Design review of the part built by this model. Coordinates are the model's own, in mm. Face numbers are marked on the shaded views. Coordinates: 2 decimals unless noted, no trailing zeros. Loops run counter-clockwise (first coordinate to the right, second up) from the corner with the lowest first, then second, coordinate; pieces in that order, holes last. Notation, with made-up numbers: (-28.75, 56.25) - (-16.75, 56.25) arc R33 cw to (-16.75, 86.25) - close; hole circle Ø8 at (-12, 46.5). An arc over 180 degrees is marked (long way). Use one line per item in the form item = value. Start each with the question number.
(1) Add section A-A (x = 34.5). State the section outline as (y, z) points.
(2) Add section B-B (z = -11). State the section outline as (x, y) points, plus the area to 3 significant figures.
(3) Clearance check with flat-ended pins moving along their axes: pin 1 Ø1.5 at (y, z) = (1, 3.5) entering from -X; pin 2 Ø2 at (y, z) = (1.5, -18.5) entering from +X; pin 3 Ø2 at (x, z) = (20, -1) entering from +Y. State where each tip first meets the part, or that it passes through.
(4) For L1, parallel to X at y = 0.5, z = -39.5; L2, parallel to X at y = 1.75, z = -16; L3, parallel to Y at x = 17, z = 2, list the stretches that pass through material, from the lowest coordinate up.
(5) The part is to be moulded in two halves that separate along X. For the marked faces 1 and 2, say which applies: pulls with the +X half, pulls with the -X half, needs draft (parallel to the pull), parting line crosses it, or undercut.
(6) Add section D-D (x = 4). State the section outline as (y, z) points, plus the area to 3 significant figures.
(7) Add section C-C (y = 2.75). State the section outline as (x, z) points (3 decimals).
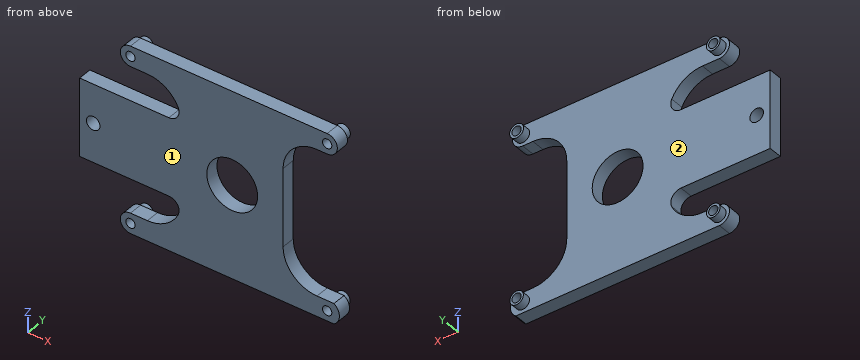
```python
from build123d import *

# Parameters (mm, degrees)
SKETCH2_R           = 1.375
SKETCH2_R_2         = 7.5
BOSS_EXTRUDE1_DEPTH = 4
SKETCH3_R           = 2
CUT_EXTRUDE1_DEPTH  = 10
SKETCH7_R           = 1.995105634
SKETCH7_R_2         = 1.375
SKETCH7_R_3         = 2.001880143
SKETCH7_R_4         = 2.050219115
SKETCH7_R_5         = 2.002328612
BOSS_EXTRUDE2_DEPTH = 2.4


with BuildPart() as part:
    # Sketch2 → Boss-Extrude1 (new body)
    with BuildSketch(Plane(origin=(0, 0, 0), x_dir=(1, 0, 0), z_dir=(0, 1, 0))):
        with BuildLine():
            Line((43.240356283, 42.558742845), (-16.759643717, 42.558742845))
            ThreePointArc((-16.759643717, 42.558742845), (-19.759643717, 39.558742845), (-16.759643717, 36.558742845))
            Line((-16.759643717, 36.558742845), (-11.759643717, 36.558742845))
            ThreePointArc((-11.759643717, 36.558742845), (-6.414418879, 35.010285392), (-2.724564688, 30.84445713))
            ThreePointArc((-2.724564688, 30.84445713), (-2.899625633, 27.955175393), (-5.435088397, 26.558742845))
            Line((-5.435088397, 26.558742845), (-28.759643717, 26.558742845))
            Line((-28.759643717, 26.558742845), (-31.759643717, 26.558742845))
            Line((-31.759643717, 26.558742845), (-31.759643717, 23.558742845))
            Line((-31.759643717, 23.558742845), (-31.759643717, 6.558742845))
            Line((-31.759643717, 6.558742845), (-31.759643717, 3.558742845))
            Line((-31.759643717, 3.558742845), (-28.759643717, 3.558742845))
            Line((-28.759643717, 3.558742845), (-5.435088397, 3.558742845))
            ThreePointArc((-5.435088397, 3.558742845), (-2.899625633, 2.162310296), (-2.724564688, -0.726971441))
            ThreePointArc((-2.724564688, -0.726971441), (-6.414418879, -4.892799703), (-11.759643717, -6.441257155))
            Line((-11.759643717, -6.441257155), (-16.759643717, -6.441257155))
            ThreePointArc((-16.759643717, -6.441257155), (-19.759643717, -9.441257155), (-16.759643717, -12.441257155))
            Line((-16.759643717, -12.441257155), (41.240356283, -12.441257155))
            ThreePointArc((41.240356283, -12.441257155), (44.240356283, -9.441257155), (41.240356283, -6.441257155))
            Line((41.240356283, -6.441257155), (38.240356283, -6.441257155))
            ThreePointArc((38.240356283, -6.441257155), (31.169288471, -3.512324967), (28.240356283, 3.558742845))
            Line((28.240356283, 3.558742845), (28.240356283, 26.558742845))
            ThreePointArc((28.240356283, 26.558742845), (31.169288471, 33.629810657), (38.240356283, 36.558742845))
            Line((38.240356283, 36.558742845), (43.240356283, 36.558742845))
            ThreePointArc((43.240356283, 36.558742845), (44.845907558, 39.558742845), (43.240356283, 42.558742845))
        make_face()
        with Locations((-16.759643717, -9.441257155)):
            Circle(SKETCH2_R, mode=Mode.SUBTRACT)
        with Locations((41.240356283, -9.441257155)):
            Circle(SKETCH2_R, mode=Mode.SUBTRACT)
        with Locations((13.240356283, 15.058742845)):
            Circle(SKETCH2_R_2, mode=Mode.SUBTRACT)
        with Locations((-16.759643717, 39.558742845)):
            Circle(SKETCH2_R, mode=Mode.SUBTRACT)
        with Locations((41.240356283, 39.558742845)):
            Circle(SKETCH2_R, mode=Mode.SUBTRACT)
    extrude(amount=BOSS_EXTRUDE1_DEPTH)

    # Sketch3 → Cut-Extrude1 (cut)
    with BuildSketch(Plane(origin=(0, 4, 0), x_dir=(1, 0, 0), z_dir=(0, 1, 0))):
        with Locations((-27.759643717, 15.058742845)):
            Circle(SKETCH3_R)
    extrude(amount=-CUT_EXTRUDE1_DEPTH, mode=Mode.SUBTRACT)

    # Sketch7 → Boss-Extrude2 (add)
    with BuildSketch(Plane(origin=(0, 4, 0), x_dir=(1, 0, 0), z_dir=(0, 1, 0))):
        with Locations((-16.759643717, 39.558742845)):
            Circle(SKETCH7_R)
        with Locations((-16.759643717, 39.558742845)):
            Circle(SKETCH7_R_2, mode=Mode.SUBTRACT)
        with Locations((-16.759643717, -9.441257155)):
            Circle(SKETCH7_R_3)
        with Locations((-16.759643717, -9.441257155)):
            Circle(SKETCH7_R_2, mode=Mode.SUBTRACT)
        with Locations((41.240356283, -9.441257155)):
            Circle(SKETCH7_R_4)
        with Locations((41.240356283, -9.441257155)):
            Circle(SKETCH7_R_2, mode=Mode.SUBTRACT)
        with Locations((41.240356283, 39.558742845)):
            Circle(SKETCH7_R_5)
        with Locations((41.240356283, 39.558742845)):
            Circle(SKETCH7_R_2, mode=Mode.SUBTRACT)
    extrude(amount=BOSS_EXTRUDE2_DEPTH)


solid = part.part
```
Computed values:
q1.outline = (0, -42.56) - (4, -42.56) - (4, -35.83) - (0, -35.83) - close; (0, 5.72) - (4, 5.72) - (4, 12.44) - (0, 12.44) - close
q2.outline = (-31.76, 0) - (6.93, 0) - (6.93, 4) - (-31.76, 4) - close; (19.55, 0) - (28.24, 0) - (28.24, 4) - (19.55, 4) - close
q2.area = 190 mm^2
q3.pin_1 = -5.51
q3.pin_2 = 28.24
q3.pin_3 = 4
q4.L1 = -19.76 to -18.13, -15.39 to 39.87, 42.61 to 44.85
q4.L2 = -31.76 to -29.52, -25.99 to 5.8, 20.68 to 28.24
q4.L3 = 0 to 4
q5.face_1 = needs draft
q5.face_2 = undercut
q6.outline = (0, -42.56) - (4, -42.56) - (4, 12.44) - (0, 12.44) - close
q6.area = 220 mm^2
q7.outline = (-31.76, -26.559) - (-5.435, -26.559) arc R3 cw to (-2.725, -30.844) arc R10 cw to (-11.76, -36.559) - (-16.76, -36.559) arc R3 ccw to (-16.76, -42.559) - (43.24, -42.559) arc R3.606 ccw to (43.24, -36.559) - (38.24, -36.559) arc R10 cw to (28.24, -26.559) - (28.24, -3.559) arc R10 cw to (38.24, 6.441) - (41.24, 6.441) arc R3 ccw to (41.24, 12.441) - (-16.76, 12.441) arc R3 ccw to (-16.76, 6.441) - (-11.76, 6.441) arc R10 cw to (-2.725, 0.727) arc R3 cw to (-5.435, -3.559) - (-31.76, -3.559) - close; hole circle Ø4 at (-27.76, -15.059); hole circle Ø2.75 at (-16.76, -39.559); hole circle Ø2.75 at (-16.76, 9.441); hole circle Ø15 at (13.24, -15.059); hole circle Ø2.75 at (41.24, -39.559); hole circle Ø2.75 at (41.24, 9.441)
